Read the model definition and answer for the solid it produces. Units are mm, in the model's axes. A direction names the side the tool comes from. Round coordinates to 2 decimals unless told otherwise and drop trailing zeros. Order: outer loops, then holes, each group sorted by start corner. A loop starts at its lowest first (then second) coordinate and runs counter-clockwise, first axis right, second up.
from build123d import *

# Parameters (mm, degrees)
ESQUISSE1_W             = 52
ESQUISSE1_H             = 40
BOSS_EXTRU_1_DEPTH      = 40
ESQUISSE2_R             = 14
ENL_V_MAT_EXTRU_1_DEPTH = 40
ESQUISSE3_R             = 3
ENL_V_MAT_EXTRU_2_DEPTH = 10
CHANFREIN1_SIZE         = 11
ESQUISSE4_R             = 3
ENL_V_MAT_EXTRU_3_DEPTH = 10


with BuildPart() as part:
    # Esquisse1 → Boss.-Extru.1 (new body)
    with BuildSketch(Plane.XY):
        with Locations((26, 20)):
            Rectangle(ESQUISSE1_W, ESQUISSE1_H)
    extrude(amount=BOSS_EXTRU_1_DEPTH)

    # Esquisse2 → Enlèv. mat.-Extru.1 (cut)
    with BuildSketch(Plane.XY.offset(40)):
        with Locations((26, 20)):
            Circle(ESQUISSE2_R)
    extrude(amount=-ENL_V_MAT_EXTRU_1_DEPTH, mode=Mode.SUBTRACT)

    # Esquisse3 → Enlèv. mat.-Extru.2 (cut)
    with BuildSketch(Plane.XY.offset(40)):
        with Locations((7, 20)):
            Circle(ESQUISSE3_R)
        with Locations((12.564971157, 33.435028843)):
            Circle(ESQUISSE3_R)
        with Locations(Location((12.564971157, 6.564971157, 0), (0, 0, 180))):
            Circle(ESQUISSE3_R)
        with Locations((39.435028843, 6.564971157)):
            Circle(ESQUISSE3_R)
        with Locations(Location((39.435028843, 33.435028843, 0), (0, 0, 180))):
            Circle(ESQUISSE3_R)
        with Locations(Location((45, 20, 0), (0, 0, 180))):
            Circle(ESQUISSE3_R)
    extrude(amount=-ENL_V_MAT_EXTRU_2_DEPTH, mode=Mode.SUBTRACT)

    # Chanfrein1
    chanfrein1_edges = [part.edges().sort_by_distance(p)[0] for p in [
        (0, 40, 20),
        (52, 40, 20),
    ]]
    chamfer(chanfrein1_edges, length=CHANFREIN1_SIZE)

    # Esquisse4 → Enlèv. mat.-Extru.3 (cut)
    with BuildSketch(Plane.XZ):
        with Locations(Location((6, 32, 0), (0, 0, 270))):
            Circle(ESQUISSE4_R)
        with Locations(Location((6, 8, 0), (0, 0, 90))):
            Circle(ESQUISSE4_R)
        with Locations(Location((46, 8, 0), (0, 0, 270))):
            Circle(ESQUISSE4_R)
        with Locations(Location((46, 32, 0), (0, 0, 90))):
            Circle(ESQUISSE4_R)
    extrude(amount=-ENL_V_MAT_EXTRU_3_DEPTH, mode=Mode.SUBTRACT)


solid = part.part
Q1. Straight lines are drawn through the part: probe 1 along X at (y, z) = (2.75, 8); probe 2 along X at (y, z) = (9, 34); probe 3 along Y at (x, z) = (26, 14). For each, find the intervals that lie inside material, in ascending order.
Outcome:
probe 1: x = 0 to 3, 9 to 43, 49 to 52
probe 2: x = 0 to 3.76, 8.24 to 10.81, 14.32 to 17.34, 34.66 to 37.68, 41.19 to 43.76, 48.24 to 52
probe 3: y = 0 to 6, 34 to 40
Q2. Flat-ended cylindrical pins translate along their axes: pin 1 (5 mm diameter, centred on x = 46, z = 8, fed in from +Y); pin 2 (8 mm diameter, centred on x = 46, z = 13, fed in from +Y); pin 3 (1.8 mm diameter, centred on x = 6.5, y = 19, fed in from +Z). Find the tip coordinate at first contact, or state that the pin passes through.
Outcome:
pin 1: stops at y = 37.5
pin 2: stops at y = 39
pin 3: stops at z = 30
Q3. A cutting plane is placed at C-C, the plane y = 8. Give the vertices of the cut face in (x, z), plus the area to 3 significant figures.
Outcome:
outline: (0, 0) - (18.79, 0) - (18.79, 40) - (15.2, 40) - (15.2, 30) - (9.93, 30) - (9.93, 40) - (0, 40) - close; (33.21, 0) - (52, 0) - (52, 40) - (42.07, 40) - (42.07, 30) - (36.8, 30) - (36.8, 40) - (33.21, 40) - close; hole circle Ø6 at (6, 8); hole circle Ø6 at (6, 32); hole circle Ø6 at (46, 8); hole circle Ø6 at (46, 32)
area: 1,280 mm2
Q4. A cutting plane is placed at D-D, the plane z = 27. Give the vertices of the cut face in (x, y).
Outcome:
outline: (0, 0) - (52, 0) - (52, 29) - (41, 40) - (11, 40) - (0, 29) - close; hole circle Ø28 at (26, 20)
Q5. A cutting plane is placed at B-B, the plane x = 26. Give the vertices of the cut face in (y, z), plus the area to 3 significant figures.
Outcome:
outline: (0, 0) - (6, 0) - (6, 40) - (0, 40) - close; (34, 0) - (40, 0) - (40, 40) - (34, 40) - close
area: 480 mm2
Q6. For a pull along X with two mould halves and no side action, classify faces 1 (the face through (5.1, 4.93, 10.86)), 2 (the face through (20, 7, 0)), 3 (the face through (52, 14, 20)), 4 (the face through (6, 35, 20)) as released by +X, released by -X, zero draft, split by the parting line, or undercut.
Outcome:
face 1: undercut
face 2: zero draft
face 3: released by +X
face 4: released by -X
Q7. A cutting plane is placed at A-A, the plane y = 20. Give the vertices of the cut face in (x, z).
Outcome:
outline: (0, 0) - (12, 0) - (12, 40) - (10, 40) - (10, 30) - (4, 30) - (4, 40) - (0, 40) - close; (40, 0) - (52, 0) - (52, 40) - (48, 40) - (48, 30) - (42, 30) - (42, 40) - (40, 40) - close
Q8. For faces 5 (the face through (43.97, 4.93, 29.79)), 6 (the face through (45, 20, 30)), 7 (the face through (26, 0, 20)), determine the directions among +Z, -Z, +X, -X, +Y, -Y from which every point of the face is accessible in a straight line to the end or side of a thin tool.
Outcome:
face 5: -Y
face 6: +Z
face 7: +Z, -Z, +X, -X, -Y
